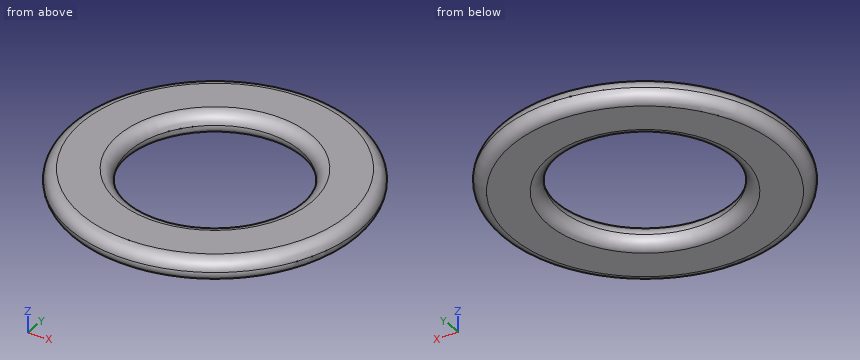
```python
from build123d import *

# Parameters (mm, degrees)
F0_R     = 12.72999994
F0_R_2   = 7.5
F1_DEPTH = 2
F2_R     = 0.99999
F3_R     = 0.99999


# Not quite as in the source:
# - a fillet or chamfer is up to 0.001 mm smaller than in the source, because OpenCascade refuses the exact size


with BuildPart() as f1:
    # F0 (on Top) → F1 (new body)
    with BuildSketch(Plane.XY):
        Circle(F0_R)
        Circle(F0_R_2, mode=Mode.SUBTRACT)
    extrude(amount=F1_DEPTH)

    # F2 (radius 1 in the source; OpenCascade refuses exactly that, so slightly less here)
    f2_edges = [f1.edges().sort_by_distance(p)[0] for p in [
        (12.73, 0, 1),
        (-12.73, 0, 0),
        (-12.73, 0, 2),
    ]]
    fillet(f2_edges, radius=F2_R)

    # F3 (radius 1 in the source; OpenCascade refuses exactly that, so slightly less here)
    f3_edges = [f1.edges().sort_by_distance(p)[0] for p in [
        (7.5, 0, 1),
        (-7.5, 0, 0),
        (-7.5, 0, 2),
    ]]
    fillet(f3_edges, radius=F3_R)


solid = f1.part
```
Read the model definition and answer for the solid it produces. Units are mm, in the model's axes. Coordinates: 2 decimals unless noted, no trailing zeros. Write each loop counter-clockwise with the first axis right and the second up, starting at its lowest first coordinate (ties: lowest second). Pieces come first, ordered by that corner, then holes. Notation, with made-up numbers: (34.25, 6) - (51.25, 6) arc R5 ccw to (51.25, 14) - close; hole circle Ø8 at (26, 45). An arc over 180 degrees is marked (long way). Answer as a JSON object with one key per item and string values. Group by question number.
1. A cutting plane is placed at C-C (z = 0.4). Determine the outline of the cut face in (x, y), plus the area to 3 significant figures.
2. Consider L1, parallel to Y at x = 0, z = 1; L2, parallel to X at y = 1, z = 0.6; L3, parallel to X at y = -6.5, z = 1. Determine where each line is inside the solid, lowest interval first. Write a range as [from, to].
3. Each of these flat-tipped pins is pushed along its axis until it touches: P1, Ø12, axis at x = -5.5, y = 10, coming from the -Z side; P2, Ø13.5, axis at x = 0, y = 0, coming from the -Z side. Where does it stop, or does it pass through?
Worked out:
{
 "1": {"outline": "circle Ø25.06 at (0, 0); hole circle Ø15.4 at (0, 0)", "area": "307 mm²"},
 "2": {"L1": "y = [-12.73, -7.5], [7.5, 12.73]", "L2": "x = [-12.61, -7.52], [7.52, 12.61]", "L3": "x = [-10.95, -3.74], [3.74, 10.95]"},
 "3": {"P1": "stops at z = 0", "P2": "passes through"}
}
